```python
from build123d import *

# Parameters (mm, degrees)
F0_W      = 35.4838
F0_H      = 31.496
F0_R      = 1.524
F1_DEPTH  = 1.4986
F2_W      = 9.8552
F2_H      = 20.2438
F3_DEPTH  = 8.4582
F2_W_2    = 5.7912
F2_H_2    = 14.9098
F2_W_3    = 4.3688
F2_H_3    = 13.4874
F4_DEPTH  = 7.0866
F2_R      = 1.4605
F5_DEPTH  = 7.6708
F6_R      = 1.4605
F2_R_2    = 0.3429
F7_DEPTH  = 8.5344
F8_DEPTH  = 8.5344
F2_W_4    = 2.3876
F2_H_4    = 10.2616
F9_DEPTH  = 2.54
F2_W_5    = 10.2616
F2_H_5    = 2.3876
F10_DEPTH = 2.54


with BuildPart() as f1:
    # F0 (on Top) → F1 (new body)
    with BuildSketch(Plane.XY):
        Rectangle(F0_W, F0_H)
        with Locations((-15.2146, -13.1445)):
            Circle(F0_R, mode=Mode.SUBTRACT)
        with Locations((15.2146, -13.1445)):
            Circle(F0_R, mode=Mode.SUBTRACT)
        with Locations((-15.2146, 13.1445)):
            Circle(F0_R, mode=Mode.SUBTRACT)
        with Locations((15.2146, 13.1445)):
            Circle(F0_R, mode=Mode.SUBTRACT)
    extrude(amount=F1_DEPTH)

    # F2 (on face) → F3 (join)
    with BuildSketch(Plane.XY.offset(1.4986)):
        with Locations((-3.7719, 4.1529)):
            Rectangle(F2_W, F2_H)
    extrude(amount=F3_DEPTH)

    # F2 (on face) → F4 (join)
    with BuildSketch(Plane.XY.offset(1.4986)):
        with Locations((4.5847, 5.9309)):
            Rectangle(F2_W_2, F2_H_2)
        with Locations((4.5847, 5.9309)):
            Rectangle(F2_W_3, F2_H_3, mode=Mode.SUBTRACT)
    extrude(amount=F4_DEPTH)

    # F2 (on face) → F5 (join)
    with BuildSketch(Plane.XY.offset(1.4986)):
        with Locations((11.7856, -4.1529)):
            Circle(F2_R)
        with Locations((11.7856, 0.300567)):
            Circle(F2_R)
        with Locations((11.7856, 4.754033)):
            Circle(F2_R)
        with Locations((11.7856, 9.2075)):
            Circle(F2_R)
    extrude(amount=F5_DEPTH)

    # F6
    f6_edges = [f1.edges().sort_by_distance(p)[0] for p in [
        (10.3251, -4.1529, 9.1694),
        (10.3251, 0.300567, 9.1694),
        (10.3251, 4.754033, 9.1694),
        (10.3251, 9.2075, 9.1694),
    ]]
    fillet(f6_edges, radius=F6_R)

    # F2 (on face) → F7 (join)
    with BuildSketch(Plane.XY.offset(1.4986)):
        with Locations((-11.1887, 1.4097)):
            Circle(F2_R_2)
        with Locations((-11.1887, 3.8989)):
            Circle(F2_R_2)
        with Locations((-11.1887, 6.3881)):
            Circle(F2_R_2)
        with Locations((-11.1887, 8.8773)):
            Circle(F2_R_2)
    extrude(amount=F7_DEPTH)

    # F2 (on face) → F8 (join)
    with BuildSketch(Plane.XY.offset(1.4986)):
        with Locations((-8.0518, -10.414)):
            Circle(F2_R_2)
        with Locations((-5.5626, -10.414)):
            Circle(F2_R_2)
        with Locations((-3.0734, -10.414)):
            Circle(F2_R_2)
        with Locations((-0.5842, -10.414)):
            Circle(F2_R_2)
    extrude(amount=F8_DEPTH)

    # F2 (on face) → F9 (join)
    with BuildSketch(Plane.XY.offset(1.4986)):
        with Locations((-11.1887, 5.1435)):
            Rectangle(F2_W_4, F2_H_4)
        with Locations((-11.1887, 1.4097)):
            Circle(F2_R_2, mode=Mode.SUBTRACT)
        with Locations((-11.1887, 3.8989)):
            Circle(F2_R_2, mode=Mode.SUBTRACT)
        with Locations((-11.1887, 6.3881)):
            Circle(F2_R_2, mode=Mode.SUBTRACT)
        with Locations((-11.1887, 8.8773)):
            Circle(F2_R_2, mode=Mode.SUBTRACT)
    extrude(amount=F9_DEPTH)

    # F2 (on face) → F10 (join)
    with BuildSketch(Plane.XY.offset(1.4986)):
        with Locations((-4.318, -10.414)):
            Rectangle(F2_W_5, F2_H_5)
        with Locations((-8.0518, -10.414)):
            Circle(F2_R_2, mode=Mode.SUBTRACT)
        with Locations((-5.5626, -10.414)):
            Circle(F2_R_2, mode=Mode.SUBTRACT)
        with Locations((-3.0734, -10.414)):
            Circle(F2_R_2, mode=Mode.SUBTRACT)
        with Locations((-0.5842, -10.414)):
            Circle(F2_R_2, mode=Mode.SUBTRACT)
    extrude(amount=F10_DEPTH)


solid = f1.part
```
Can you work these out from the model? Positions are in its coordinate system, mm. A direction names the side the tool comes from. Give positions to 0.01 mm unless a question says otherwise; leave off trailing zeros. Loops run counter-clockwise (first coordinate to the right, second up) from the corner with the lowest first, then second, coordinate; pieces in that order, holes last. Notation, with made-up numbers: M 45.5,85.5 L 86.5,85.5 A21 ccw 86.5,96.5 Z; hole C 4,-27.5 d11. An arc over 180 degrees is marked long. Use one line per item in the form item = value. Start each with the question number.
(1) Please list where these lines run through material, in increasing order: line 1 (X direction, y = 11.5, z = 4.5); line 2 (X direction, y = 3.5, z = 8); line 3 (Y direction, x = 16, z = 1.25).
(2) I want a section at A-A, the plane z = 3. State how many separate pieces and enclosed holes the cut face has, and give its area (3 significant figures).
(3) I want a section at C-C, the plane y = -12.5. Write out the boundary of the cut face in (x, z), and give its area (3 significant figures).
(4) I want a section at B-B, the plane x = -6.5. Write out the boundary of the cut face in (y, z).
(5) I'm going to push flat-ended pins straight in: P1, Ø1.3, axis at x = 3.5, z = 5, coming from the -Y side; P2, Ø5.5, axis at y = 3.5, z = 5, coming from the -X side; P3, Ø4, axis at x = -15.21, y = -13.14, coming from the -Z side; P4, Ø4, axis at x = 15.21, y = -13.14, coming from the +Z side. Where does each tip first touch, or does it pass through?
(6) On a 3-axis mill with a long thin cutter (end or side, diameter ignored), from which of +Z, -Z, +X, -X, +Y, -Y can I reach the whole of each face in a straight line? I mean faces 1 (the flat face through (-11, 5, 4.039)), 2 (the flat face through (0.813, -10, 3)), 3 (the flat face through (-4, -9.22, 3)). Say none if no direction works.
Worked out:
q1.line_1 = -8.7 to 1.16, 1.69 to 2.4, 6.77 to 7.48
q1.line_2 = -8.7 to 1.16, 1.69 to 2.4, 6.77 to 7.48, 11.1 to 12.48
q1.line_3 = -15.75 to -14.45, -11.84 to 11.84, 14.45 to 15.75
q2.separate_pieces = 8
q2.enclosed_holes = 1
q2.area = 303 mm²
q3.outline = M -17.74,0 L -16.6,0 L -16.6,1.5 L -17.74,1.5 Z; M -13.83,0 L 13.83,0 L 13.83,1.5 L -13.83,1.5 Z; M 16.6,0 L 17.74,0 L 17.74,1.5 L 16.6,1.5 Z
q3.area = 44.9 mm²
q4.outline = M -15.75,0 L 15.75,0 L 15.75,1.5 L 14.27,1.5 L 14.27,9.96 L -5.97,9.96 L -5.97,1.5 L -9.22,1.5 L -9.22,4.04 L -11.61,4.04 L -11.61,1.5 L -15.75,1.5 Z
q5.P1 = -1.52
q5.P2 = -12.38
q5.P3 = 0
q5.P4 = 1.5
q6.face_1 = +Z
q6.face_2 = +Z, +X, -Y
q6.face_3 = +Z, +X, -X
